Read the model definition and answer for the solid it produces. Units are mm, in the model's axes. A direction names the side the tool comes from. Give positions to 0.01 mm unless a question says otherwise; leave off trailing zeros. Loops run counter-clockwise (first coordinate to the right, second up) from the corner with the lowest first, then second, coordinate; pieces in that order, holes last. Notation, with made-up numbers: (66.5, 45) -> (116.5, 45) arc R16 cw to (116.5, 52) -> close; hole circle Ø10 at (15.25, 75.25). An arc over 180 degrees is marked (long way). Answer as CSV lines item,"result". Start each with the question number.
```python
from build123d import *

# Parameters (mm, degrees)
BOSS_EXTRUDE1_DEPTH = 13.716
SCALE1_SCALE        = 1.5


with BuildPart() as part:
    # Sketch1 → Boss-Extrude1 (new body)
    with BuildSketch(Plane(origin=(0, 0, 0), x_dir=(1, 0, 0), z_dir=(0, 1, 0))):
        with BuildLine():
            Line((33.911483948, -31.607658541), (48.863023265, 19.10634644))
            Line((48.863023265, 19.10634644), (19.060968545, -7.15987128))
            ThreePointArc((19.060968545, -7.15987128), (15.22639693, -18.310469683), (16.13127503, -6.553727794))
            Line((16.13127503, -6.553727794), (3.778414078, 36.56159637))
            Line((3.778414078, 36.56159637), (-8.574446874, -6.553727794))
            ThreePointArc((-8.574446874, -6.553727794), (-7.669568774, -18.310469683), (-11.504140389, -7.15987128))
            Line((-11.504140389, -7.15987128), (-41.306195109, 19.10634644))
            Line((-41.306195109, 19.10634644), (-26.354655792, -31.607658541))
            Line((-26.354655792, -31.607658541), (33.911483948, -31.607658541))
        make_face()
    extrude(amount=BOSS_EXTRUDE1_DEPTH)


with BuildPart() as part_1:
    # Scale1: scaled about (3.778414078, 6.858, 9.196569952)
    add(part.part.scale(SCALE1_SCALE).moved(Location((-1.889207039, -3.429, -4.598284976))))


solid = part_1.part
```
(1) The mould has two halves that part along X. Classify faces 1 (the face through (3, -3.429, 2)), 2 (the face through (60.035, 6.714, 5.31)), 3 (the face through (21.305, 6.714, 22.933)): pulls with the +X half, pulls with the -X half, needs draft (parallel to the pull), parting line crosses it, or undercut.
(2) Find the intervals of material crossed by line 1 along X through (y, z) = (15.25, -32.5); line 2 along X through (y, z) = (4, -31); line 3 along X through (y, z) = (3, -46.5), in increasing order. Write a range as from..to.
(3) Each of these flat-tipped pins is pushed along its axis until it touches: P1, Ø8, axis at y = 4.5, z = 12, coming from the +X side; P2, Ø3, axis at y = 0, z = 27.5, coming from the -X side; P3, Ø23, axis at x = -15.2, z = 14.14, coming from the -Y side; P4, Ø5, axis at y = -1.5, z = 18.5, coming from the -X side. Where does it stop, or does it pass through?
(4) A tool of negligible diameter and unlimited length cuts with its end or side. For faces 4 (the face through (3, 17.145, 2)), 5 (the face through (13.173, 6.714, -26.651)), from which of +Z, -Z, +X, -X, +Y, -Y can it reach the whole face along a straight path? Write none if from no direction.
(5) Find section D-D on x = -43. Write down the section's boundary in (y, z) (3 decimals), then the cut area to 3 significant figures.
(6) Find section A-A on z = -29. Write down the section's boundary in (x, y) (3 decimals).
(7) Find section C-C on z = 1.5. Write down the section's boundary in (x, y) (3 decimals).
(8) Find section B-B on y = 9.25. Write down the section's boundary in (x, z), then the cut area to 3 significant figures.
Answer block:
1,face 1,"needs draft"
1,face 2,"pulls with the +X half"
1,face 3,"undercut"
2,line 1,"x = -63.63..-62.99, -3.94..11.5, 70.55..71.18"
2,line 2,"x = -63.18..-61.29, -4.37..11.93, 68.84..70.74"
2,line 3,"x = 0.07..7.49"
3,P1,"stops at x = 59.24"
3,P2,"stops at x = -46.38"
3,P3,"stops at y = -3.43"
3,P4,"stops at x = -49.33"
4,face 4,"+Z, -Z, +X, -X, +Y"
4,face 5,"-Z, +Y, -Y"
5,outline,"(-3.429, -14.883) -> (17.145, -14.883) -> (17.145, 37.458) -> (-3.429, 37.458) -> close"
5,area,"1,080 mm2"
6,outline,"(-62.593, -3.429) -> (-59.018, -3.429) -> (-59.018, 17.145) -> (-62.593, 17.145) -> close; (-4.943, -3.429) -> (12.5, -3.429) -> (12.5, 17.145) -> (-4.943, 17.145) -> close; (66.574, -3.429) -> (70.15, -3.429) -> (70.15, 17.145) -> (66.574, 17.145) -> close"
7,outline,"(-53.601, -3.429) -> (-24.412, -3.429) -> (-24.412, 17.145) -> (-53.601, 17.145) -> close; (-13.682, -3.429) -> (21.238, -3.429) -> (21.238, 17.145) -> (-13.682, 17.145) -> close; (31.969, -3.429) -> (61.158, -3.429) -> (61.158, 17.145) -> (31.969, 17.145) -> close"
8,outline,"(-63.85, -33.26) -> (-19.15, 6.14) arc R8.92 cw (long way) to (-14.75, 5.23) -> (3.78, -59.44) -> (22.31, 5.23) arc R8.92 cw (long way) to (26.7, 6.14) -> (71.41, -33.26) -> (48.98, 42.81) -> (-41.42, 42.81) -> close"
8,area,"5,750 mm2"
